The listing builds one solid part. Answer for the finished solid, in the listing's coordinates (mm). A direction names the side the tool comes from. Give positions to 0.01 mm unless a question says otherwise; leave off trailing zeros. Order: outer loops, then holes, each group sorted by start corner. A loop starts at its lowest first (then second) coordinate and runs counter-clockwise, first axis right, second up. Notation, with made-up numbers: (28, 83.5) - (44, 83.5) arc R20 cw to (44, 121.5) - close; hole circle Ø6 at (42, 60). An arc over 180 degrees is marked (long way). Answer as a JSON object with one key per item and string values. Group by question number.
Q1. A cutting plane is placed at C-C, the plane x = 31. Give the vertices of the cut face in (y, z), and give its area (3 significant figures).
Q2. Consider line 1 (X direction, y = 5.65, z = 53.25); line 2 (Z direction, x = -10, y = 27); line 3 (X direction, y = 11.75, z = 55.5). Determine where each line is inside the solid, lowest interval first.
Q3. For faces 5 (the face through (44.6, 26.43, 53.87)), 6 (the face through (57, 22, 54)), 7 (the face through (39.883, 4.309, 59.549)), determine the directions among +Z, -Z, +X, -X, +Y, -Y from which every point of the face is accessible in a straight line to the end or side of a thin tool.
Q4. The mould has two halves that part along X. Classify faces 1 (the face through (20.927, 16.155, 55.395)), 2 (the face through (12.536, 14.092, 53.874)), 3 (the face through (20, 9, 63)), 4 (the face through (49.4, 0.57, 53.87)): released by +X, released by -X, zero draft, split by the parting line, or undercut.
Q5. A cutting plane is placed at A-A, the plane x = 5.65. Give the vertices of the cut face in (y, z).
Q6. A cutting plane is placed at B-B, the plane z = 60.5. Give the vertices of the cut face in (x, y), and give its area (3 significant figures).
Q7. Given pin 1 (8 mm diameter, centred on x = 52.5, z = 56, fed in from +Y); pin 2 (1.2 mm diameter, centred on x = 16.5, z = 60.5, fed in from +Y); pin 3 (8 mm diameter, centred on x = 16.7, z = 55.5, fed in from -Y), each flat-ended and moving along its own axis, determine where each tip first touches the part or whether it passes through.
from build123d import *

# Parameters (mm, degrees)
SKETCH011_R     = 1.5
PAD008_DEPTH    = 18
SKETCH012_R     = 12
POCKET_DEPTH    = 3
SKETCH015_R     = 1.2
POCKET007_DEPTH = 32.651
SKETCH016_R     = 2.5
POCKET008_DEPTH = 4.5
SKETCH022_R     = 3.5
POCKET009_DEPTH = 7
SKETCH023_R     = 2.65
POCKET010_DEPTH = 5.001


with BuildPart() as part:
    # Sketch011 → Pad008 (new body)
    with BuildSketch(Plane.XY.offset(45)):
        with BuildLine():
            ThreePointArc((7.8, 12.65), (12.595297, 14.1318), (15.718671, 18.060558))
            Line((15.718671, 18.060558), (17.218671, 18.060558))
            ThreePointArc((17.218671, 18.060558), (20.988406, 16.152612), (24.873527, 17.813033))
            Line((24.873527, 17.813033), (32.510589, 26.334787))
            ThreePointArc((36, 25), (34.714555, 26.867996), (32.510589, 26.334787))
            Line((36, 25), (36, 17))
            ThreePointArc((36, 17), (40, 13), (44, 17))
            Line((44, 17), (44, 25))
            ThreePointArc((45.999998, 27), (44.585786, 26.414213), (44, 25))
            Line((45.999998, 27), (62, 27))
            ThreePointArc((62, 22), (64.5, 24.5), (62, 27))
            Line((62, 22), (52, 22))
            ThreePointArc((52, 22), (50.585786, 21.414213), (50, 20))
            Line((50, 20), (50, 2))
            ThreePointArc((48, 0), (49.414214, 0.585787), (50, 2))
            Line((-4, 0), (48, 0))
            ThreePointArc((-4, 0), (-6.828417, -1.171563), (-8, -3.999973))
            Line((-8, -3.999973), (-8, -13.999973))
            Line((-13, -13.999973), (-8, -13.999973))
            Line((-13, 32.65), (-13, -13.999973))
            Line((-8, 32.65), (-13, 32.65))
            Line((-8, 22.65), (-8, 32.65))
            ThreePointArc((-8, 22.65), (-5.071068, 15.578932), (2, 12.65))
            Line((7.8, 12.65), (2, 12.65))
        make_face()
        with Locations((36.65, 5.65)):
            Circle(SKETCH011_R, mode=Mode.SUBTRACT)
        with Locations((5.65, 5.65)):
            Circle(SKETCH011_R, mode=Mode.SUBTRACT)
    extrude(amount=PAD008_DEPTH)

    # Sketch012 → Pocket (cut)
    with BuildSketch(Plane(origin=(0, 0, 45), x_dir=(1, 0, 0), z_dir=(0, 0, -1))):
        with Locations((21.15, -21.15)):
            Circle(SKETCH012_R)
    extrude(amount=-POCKET_DEPTH, mode=Mode.SUBTRACT)

    # Sketch015 → Pocket007 (cut, through all)
    with BuildSketch(Plane(origin=(0, 0, 45), x_dir=(1, 0, 0), z_dir=(0, -1, 0))):
        with Locations((16.7, 10.5)):
            Circle(SKETCH015_R)
    extrude(amount=-POCKET007_DEPTH, mode=Mode.SUBTRACT)

    # Sketch016 → Pocket008 (cut)
    with BuildSketch(Plane(origin=(0, 0, 45), x_dir=(1, 0, 0), z_dir=(0, -1, 0))):
        with Locations((16.7, 10.5)):
            Circle(SKETCH016_R)
    extrude(amount=-POCKET008_DEPTH, mode=Mode.SUBTRACT)

    # Sketch022 → Pocket009 (cut)
    with BuildSketch(Plane.XY.offset(63)):
        with Locations((5.65, 5.65)):
            Circle(SKETCH022_R)
        with Locations((36.65, 5.65)):
            Circle(SKETCH022_R)
    extrude(amount=-POCKET009_DEPTH, mode=Mode.SUBTRACT)

    # Sketch023 → Pocket010 (cut, through all)
    with BuildSketch(Plane(origin=(-8, 0, 45), x_dir=(0, 1, 0), z_dir=(1, 0, 0))):
        with Locations((-8.499973, 9)):
            Circle(SKETCH023_R)
        with Locations((27.15, 9)):
            Circle(SKETCH023_R)
    extrude(amount=-POCKET010_DEPTH, mode=Mode.SUBTRACT)


solid = part.part
Reply:
{
 "1": {"outline": "(0, 45) - (14.3, 45) - (14.3, 48) - (24.65, 48) - (24.65, 63) - (0, 63) - close", "area": "413 mm^2"},
 "2": {"line 1": "x = -13 to 4.15, 7.15 to 35.15, 38.15 to 50", "line 2": "z = 45 to 51.35, 56.65 to 63", "line 3": "x = -13 to 15.5, 17.9 to 50"},
 "3": {"face 5": "+Z, -Z, +Y", "face 6": "+Z, -Z, +X, -Y", "face 7": "+Z"},
 "4": {"face 1": "undercut", "face 2": "undercut", "face 3": "zero draft", "face 4": "released by +X"},
 "5": {"outline": "(0, 45) - (4.15, 45) - (4.15, 56) - (2.15, 56) - (2.15, 63) - (0, 63) - close; (7.15, 45) - (12.65, 45) - (12.65, 63) - (9.15, 63) - (9.15, 56) - (7.15, 56) - close"},
 "6": {"outline": "(-13, -14) - (-8, -14) - (-8, -4) arc R4 cw to (-4, 0) - (48, 0) arc R2 ccw to (50, 2) - (50, 20) arc R2 cw to (52, 22) - (62, 22) arc R2.5 ccw to (62, 27) - (46, 27) arc R2 ccw to (44, 25) - (44, 17) arc R4 cw to (36, 17) - (36, 25) arc R2 ccw to (32.51, 26.33) - (24.87, 17.81) arc R5 cw to (17.22, 18.06) - (15.72, 18.06) arc R8.5 cw to (7.8, 12.65) - (2, 12.65) arc R10 cw to (-8, 22.65) - (-8, 32.65) - (-13, 32.65) - close; hole circle Ø7 at (5.65, 5.65); hole circle Ø7 at (36.65, 5.65)", "area": "1,250 mm^2"},
 "7": {"pin 1": "stops at y = 27", "pin 2": "stops at y = 18.06", "pin 3": "stops at y = 0"}
}
